Design review of the part built by this model. Coordinates are the model's own, in mm. Coordinates: 2 decimals unless noted, no trailing zeros. Loops run counter-clockwise (first coordinate to the right, second up) from the corner with the lowest first, then second, coordinate; pieces in that order, holes last. Notation, with made-up numbers: (-27.5, -31.5) -> (16.5, -31.5) arc R8 ccw to (16.5, -27.5) -> close; hole circle Ø2 at (57, 46). An arc over 180 degrees is marked (long way). Use a Markdown table: item, result. Add a question column.
Q1. Take a section at A-A on z = 0. Write out the cut boundary in (x, y).
Q2. For probe 1 along Y at (x, z) = (2.85, 0); probe 2 along Z at (x, y) = (4, 0); probe 3 along Y at (x, z) = (1.35, -6.5), list the stretches that pass through material, from the lowest coordinate up.
Q3. Take a section at C-C on z = -14.5. Write out the cut boundary in (x, y), plus the area to 3 significant figures.
Q4. Take a section at D-D on z = 14. Write out the cut boundary in (x, y), plus the area to 3 significant figures.
Q5. Clearance check with flat-ended pins moving along their axes: pin 1 Ø2 at (x, y) = (0.5, -9.5) entering from -Z; pin 2 Ø1 at (x, z) = (3, 2) entering from +Y. State where each tip first meets the part, or that it passes through.
Q6. Take a section at B-B on y = 14.5. Write out the cut boundary in (x, z), plus the area to 3 significant figures.
Q7. Draft analysis for pull direction Y (two halves, no side actions). For faces 1 (the face through (5.842, 4, 0)), 2 (the face through (2.88, 2.287, -15.693)), state which applies: pulls with the +Y half, pulls with the -Y half, needs draft (parallel to the pull), parting line crosses it, or undercut.
from build123d import *

# Parameters (mm, degrees)
BASPROSKE_W         = 5.842
BASPROSKE_H         = 19.05
TOOTHCUT_DEPTH      = 28.566899789
TEETHCUTS_COUNT     = 10
TEETHCUTS_ANGLE     = 324
BORSKE_R            = 2.38125
BORE_DEPTH          = 50.8000508
SKETCH1_R           = 2.5
CUT_EXTRUDE1_DEPTH  = 5.842
BOSS_EXTRUDE1_DEPTH = 5.842


with BuildPart() as part:
    # BasProSke → Base-Revolve (revolve)
    with BuildSketch(Plane(origin=(0, 0, 0), x_dir=(1, 0, 0), z_dir=(0, 1, 0)), mode=Mode.PRIVATE) as base_revolve_sk:
        with Locations((2.921, 9.525)):
            Rectangle(BASPROSKE_W, BASPROSKE_H)
    revolve(base_revolve_sk.sketch.rotate(Axis((-10, 0, 0), (1, 0, 0)), 180), axis=Axis((-10, 0, 0), (1, 0, 0)))

    # TooCutSke → ToothCut (cut, through all)
    with BuildSketch(Plane(origin=(0, 0, 0), x_dir=(0, 0, -1), z_dir=(1, 0, 0))):
        with BuildLine():
            ThreePointArc((1.873548596, 11.756630659), (0, 11.90498), (-1.873548596, 11.756630659))
            ThreePointArc((-1.873548596, 11.756630659), (-2.656568084, 15.60034376), (-5.548507123, 18.250615164))
            ThreePointArc((-5.548507123, 18.250615164), (0, 19.0754), (5.548507123, 18.250615164))
            ThreePointArc((5.548507123, 18.250615164), (2.656568084, 15.60034376), (1.873548596, 11.756630659))
        make_face()
    toothcut = extrude(amount=TOOTHCUT_DEPTH, mode=Mode.SUBTRACT)

    # TeethCuts: ToothCut ×10 about axis
    teethcuts_axis = Axis((-10, 0, 0), (1, 0, 0))
    for i in range(1, TEETHCUTS_COUNT):
        add(toothcut.rotate(teethcuts_axis, i * TEETHCUTS_ANGLE / (TEETHCUTS_COUNT - 1)), mode=Mode.SUBTRACT)

    # BorSke → Bore (cut, symmetric)
    with BuildSketch(Plane(origin=(0, 0, 0), x_dir=(0, 0, -1), z_dir=(1, 0, 0))):
        with Locations(Location((0, 0, 0), (0, 0, 180))):
            Circle(BORSKE_R)
    extrude(amount=BORE_DEPTH, both=True, mode=Mode.SUBTRACT)

    # Sketch1 → Cut-Extrude1 (cut)
    with BuildSketch(Plane(origin=(5.842, 0, 0), x_dir=(0, 0, -1), z_dir=(1, 0, 0))):
        Circle(SKETCH1_R)
    extrude(amount=-CUT_EXTRUDE1_DEPTH, mode=Mode.SUBTRACT)

    # Sketch2 → Boss-Extrude1 (add)
    with BuildSketch(Plane(origin=(5.842, 0, 0), x_dir=(0, 0, -1), z_dir=(1, 0, 0))):
        with BuildLine():
            Line((-1.5, 2), (1.5, 2))
            ThreePointArc((1.5, 2), (0, 2.5), (-1.5, 2))
        make_face()
    extrude(amount=-BOSS_EXTRUDE1_DEPTH)


solid = part.part
Answer list:
| question | item | result |
|---|---|---|
| 1 | outline | (0, -11.9) -> (5.84, -11.9) -> (5.84, -2.5) -> (0, -2.5) -> close; (0, 2) -> (5.84, 2) -> (5.84, 11.9) -> (0, 11.9) -> close |
| 2 | probe 1 | -11.9 to -2.5, 2 to 11.9 |
| 2 | probe 2 | -19.05 to -2.5, 2.5 to 19.05 |
| 2 | probe 3 | -17.51 to -12.29, -9.97 to 9.97, 12.29 to 17.51 |
| 3 | outline | (0, -11.61) -> (5.84, -11.61) -> (5.84, -7.94) -> (0, -7.94) -> close; (0, -2.42) -> (5.84, -2.42) -> (5.84, 2.42) -> (0, 2.42) -> close; (0, 7.94) -> (5.84, 7.94) -> (5.84, 11.61) -> (0, 11.61) -> close |
| 3 | area | 71.1 mm² |
| 4 | outline | (0, -11.63) -> (5.84, -11.63) -> (5.84, -7.33) -> (0, -7.33) -> close; (0, -2.41) -> (5.84, -2.41) -> (5.84, 2.41) -> (0, 2.41) -> close; (0, 7.33) -> (5.84, 7.33) -> (5.84, 11.63) -> (0, 11.63) -> close |
| 4 | area | 78.4 mm² |
| 5 | pin 1 | z = -15.58 |
| 5 | pin 2 | y = 15.31 |
| 6 | outline | (0, -7.05) -> (5.84, -7.05) -> (5.84, -2.17) -> (0, -2.17) -> close; (0, 2.17) -> (5.84, 2.17) -> (5.84, 7.05) -> (0, 7.05) -> close |
| 6 | area | 57.1 mm² |
| 7 | face 1 | needs draft |
| 7 | face 2 | undercut |
